Autodesk Inventor part; units mm, degrees
ref_plane "YZ Plane" through (0, 0, 0) normal (1, 0, 0) x (0, 1, 0)
ref_plane "XZ Plane" through (0, 0, 0) normal (0, 1, 0) x (-1, 0, 0)
ref_plane "XY Plane" through (0, 0, 0) normal (0, 0, 1) x (1, 0, 0)
sketch "Skizze1" plane through (0, 0, 0) normal (0, 1, 0) x (-1, 0, 0)
  line L0 (-2.5, 15.5) -> (2.5, 15.5)
  line L1 (2.5, 15.5) -> (2.5, -15.5)
  line L2 (2.5, -15.5) -> (-2.5, -15.5)
  line L3 (-2.5, -15.5) -> (-2.5, 15.5)
  line L4 (-2.5, 15.5) -> (2.5, -15.5) construction
  line L5 (2.5, 15.5) -> (-2.5, -15.5) construction
  circle A0 centre (0, 12.5) radius 1
  circle A1 centre (0, -12.5) radius 1
  line L6 (3.5, 0) -> (-3.5, 0)
  point P0 (0, 0)
  point P1 (0, 0)
  dimension "d1" = 5
  dimension "d2" = 3
  dimension "d3" = 2
  dimension "d9" = 25
extrude "Extrusion1" add sketch "Skizze1" along normal mid plane 1
chamfer "Fase1" distance 2 angle 45 4 edges at (-2.5, 0, 15.5) (2.5, 0, 15.5) (-2.5, 0, -15.5) (2.5, 0, -15.5)
properties part number "Schenkel"
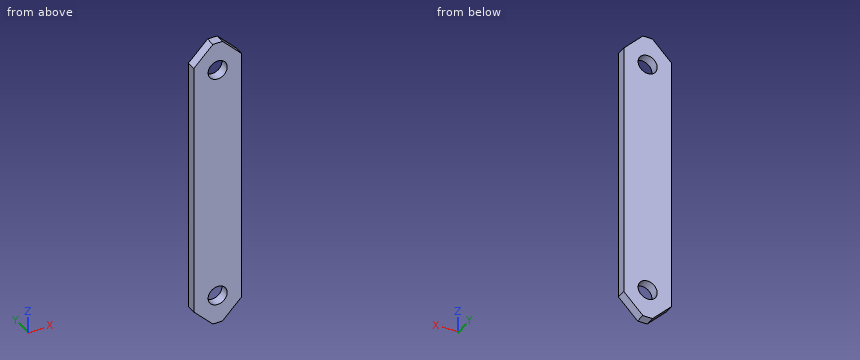
Can you work these out from the model? Positions are in its coordinate system, mm. Round coordinates to 2 decimals unless told otherwise and drop trailing zeros. Order: outer loops, then holes, each group sorted by start corner. A loop starts at its lowest first (then second) coordinate and runs counter-clockwise, first axis right, second up. Notation, with made-up numbers: (-23.5, 39.5) -> (5.5, 39.5) arc R23 cw to (5.5, 72.5) -> close; hole circle Ø9 at (-40, 13). An arc over 180 degrees is marked (long way). Write each question's results on one line, items separated by ' | '. Start each with the question number.
Item 1: Please list where these lines run through material, in increasing order: L1, parallel to Z at x = 0, y = -0.15; L2, parallel to Z at x = -0.9, y = -0.35; L3, parallel to Z at x = 2.2, y = 0.15.
Item 2: If we section it at B-B, the plane x = 0: Write out the boundary of the cut face in (y, z), then the cut area to 3 significant figures.
Item 3: If we section it at A-A, the plane z = -12.5: Write out the boundary of the cut face in (x, y).
Item 4: If we section it at C-C, the plane y = -0.15: Write out the boundary of the cut face in (x, z).
Item 5: If we section it at D-D, the plane x = 2: Write out the boundary of the cut face in (y, z), then the cut area to 3 significant figures.
Results:
1) L1: z = -15.5 to -13.5, -11.5 to 11.5, 13.5 to 15.5 | L2: z = -15.1 to -12.94, -12.06 to 12.06, 12.94 to 15.1 | L3: z = -13.8 to 13.8
2) outline: (-0.5, -15.5) -> (0.5, -15.5) -> (0.5, -13.5) -> (-0.5, -13.5) -> close; (-0.5, -11.5) -> (0.5, -11.5) -> (0.5, 11.5) -> (-0.5, 11.5) -> close; (-0.5, 13.5) -> (0.5, 13.5) -> (0.5, 15.5) -> (-0.5, 15.5) -> close | area: 27.0 mm2
3) outline: (-2.5, -0.5) -> (-1, -0.5) -> (-1, 0.5) -> (-2.5, 0.5) -> close; (1, -0.5) -> (2.5, -0.5) -> (2.5, 0.5) -> (1, 0.5) -> close
4) outline: (-2.5, -13.5) -> (-0.5, -15.5) -> (0.5, -15.5) -> (2.5, -13.5) -> (2.5, 13.5) -> (0.5, 15.5) -> (-0.5, 15.5) -> (-2.5, 13.5) -> close; hole circle Ø2 at (0, -12.5); hole circle Ø2 at (0, 12.5)
5) outline: (-0.5, -14) -> (0.5, -14) -> (0.5, 14) -> (-0.5, 14) -> close | area: 28.0 mm2
